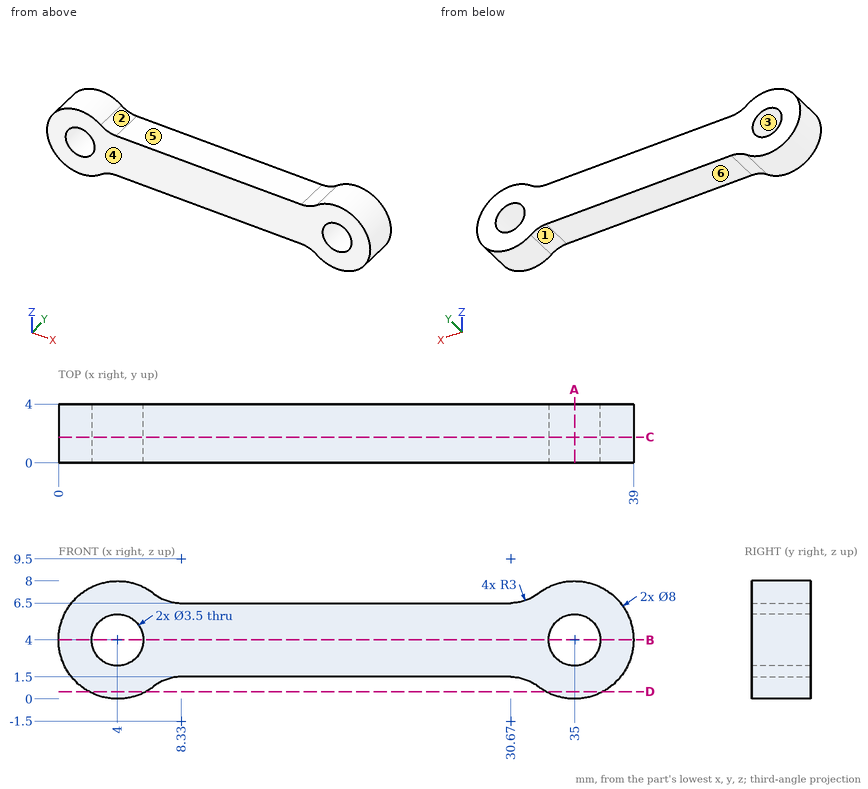
Part print with two shaded views. Sizes in mm from the minimum x, y, z corner. A direction names the side the tool comes from. Coordinates: 2 decimals unless noted, no trailing zeros. Loops run counter-clockwise (first coordinate to the right, second up) from the corner with the lowest first, then second, coordinate; pieces in that order, holes last. Notation, with made-up numbers: (85, 1) - (129, 1) arc R13 ccw to (129, 16) - close; hole circle Ø9 at (-10.5, 38.5). An arc over 180 degrees is marked (long way). Write each question's results on one line, items separated by ' | '. Start each with the question number.
Q1. Slice it at B-B on z = 4. Give the cut face in (x, y).
Q2. Slice it at D-D on z = 0.5. Give the cut face in (x, y), and give its area (3 significant figures).
Q3. Slice it at C-C on y = 1.75. Give the cut face in (x, z).
Q4. Two-plate mould, pull along Z, no slides. Class the marked faces 1, 2 and 3: +Z half, -Z half, draft (parallel to the pull), parting line (faces both ways), or undercut.
Q5. Slice it at A-A on x = 35. Give the cut face in (y, z), and give its area (3 significant figures).
Q6. Probe line 1 along X through (y, z) = (2.05, 4); line 2 along Z through (x, y) = (4, 3.15); line 3 along X through (y, z) = (0.65, 5.5). List the from-to ranges inside material, lowest first.
Q7. Drop a flat-ended pin along its axis: pin 1 Ø2 at (x, y) = (24.5, 1) entering from -Z. Give the stop position or say it passes through.
Q8. Which spindle directions (+Z, -Z, +X, -X, +Y, -Y) get a long thin tool onto all of the face, cutting with end or side? Do the marked faces 4, 5 and 6. Say none if no direction does.
Answer:
1) outline: (0, 0) - (2.25, 0) - (2.25, 4) - (0, 4) - close; (5.75, 0) - (33.25, 0) - (33.25, 4) - (5.75, 4) - close; (36.75, 0) - (39, 0) - (39, 4) - (36.75, 4) - close
2) outline: (2.06, 0) - (5.94, 0) - (5.94, 4) - (2.06, 4) - close; (33.06, 0) - (36.94, 0) - (36.94, 4) - (33.06, 4) - close | area: 31.0 mm2
3) outline: (6.47, 0.86) arc R3 cw to (8.33, 1.5) - (30.67, 1.5) arc R3 cw to (32.53, 0.86) arc R4 ccw (long way) to (32.53, 7.14) arc R3 cw to (30.67, 6.5) - (8.33, 6.5) arc R3 cw to (6.47, 7.14) arc R4 ccw (long way) to start; hole circle Ø3.5 at (4, 4); hole circle Ø3.5 at (35, 4)
4) face 1: -Z half | face 2: +Z half | face 3: undercut
5) outline: (0, 0) - (4, 0) - (4, 2.25) - (0, 2.25) - close; (0, 5.75) - (4, 5.75) - (4, 8) - (0, 8) - close | area: 18.0 mm2
6) line 1: x = 0 to 2.25, 5.75 to 33.25, 36.75 to 39 | line 2: z = 0 to 2.25, 5.75 to 8 | line 3: x = 0.29 to 3.1, 4.9 to 34.1, 35.9 to 38.71
7) pin 1: stops at z = 1.5
8) face 4: +Z, -Z, +X, -X, -Y | face 5: +Z, +Y, -Y | face 6: -Z, +Y, -Y
